Geometry: final body of the model. Coordinates: model frame, mm. Face numbers are marked on the shaded views. Give positions to 0.01 mm unless a question says otherwise; leave off trailing zeros. Order: outer loops, then holes, each group sorted by start corner. A loop starts at its lowest first (then second) coordinate and runs counter-clockwise, first axis right, second up. Notation, with made-up numbers: (-32.75, -19.75) -> (-28.75, -19.75) arc R15 cw to (-28.75, -10.75) -> close; hole circle Ø3 at (-17.75, 76.5). An arc over 180 degrees is marked (long way). Answer in a Markdown table with one row per item. Add a question column.
Q1. Line query: line 1 along X through (y, z) = (0, 3.25); line 2 along X through (y, z) = (-1, 5.5); line 3 along Y through (x, z) = (-4.25, -0.75). Output: solid intervals per line, ascending. Write a range as from..to.
Q2. Pull-direction query (X, two-part tool) for the marked faces 1, 2, 3 and 4; classes: +X half, -X half, draft (parallel to the pull), parting line (faces both ways), or undercut.
Q3. Cut plane A-A on z = 1.5. Return the cut outline in (x, y), and give its area (3 significant figures).
Q4. Contact query for flat-ended pins moving along their axis: P1, Ø5, axis at x = -3, z = -3, coming from the +Y side; P2, Ø3, axis at x = 0.5, z = 0.5, coming from the +Y side; P3, Ø7, axis at x = 0, y = 0, coming from the -Z side. Output: stop coordinate, or through.
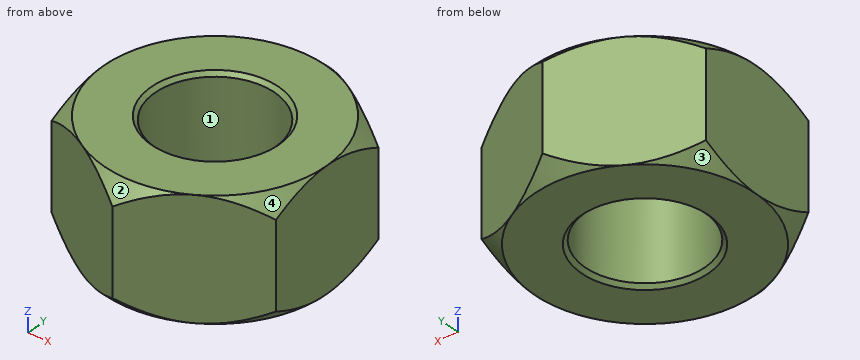
from build123d import *

# Parameters (mm, degrees)
SKETCH1_R           = 6
BOSS_EXTRUDE1_DEPTH = 6
SKETCH6_OUTSIDE_W   = 74.94
SKETCH6_OUTSIDE_H   = 78.374
SKETCH6_OUTSIDE_R   = 11.1
CUT_EXTRUDE5_DEPTH  = 21.772337374
CUT_EXTRUDE5_DRAFT  = -45
SKETCH7_OUTSIDE_W   = 74.94
SKETCH7_OUTSIDE_H   = 78.374
SKETCH7_OUTSIDE_R   = 11.1
CUT_EXTRUDE6_DEPTH  = 21.772337374
CUT_EXTRUDE6_DRAFT  = -45


with BuildPart() as part:
    # Sketch1 → Boss-Extrude1 (new, symmetric)
    with BuildSketch(Plane.XY):
        Polygon((0, -12.817175976), (11.1, -6.408587988), (11.1, 6.408587988), (0, 12.817175976), (-11.1, 6.408587988), (-11.1, -6.408587988), align=None)
        Circle(SKETCH1_R, mode=Mode.SUBTRACT)
    extrude(amount=BOSS_EXTRUDE1_DEPTH, both=True)

    # Cut-Extrude3 cone 1 section (through the dimple's axis) → Cut-Extrude3 (revolve, cut)
    with BuildSketch(Plane(origin=(0, 0, 6), x_dir=(0, -1, 0), z_dir=(1, 0, 0))):
        Polygon((0, 0), (6.381, 0), (0, 6.381), align=None)
    revolve(axis=Axis((0, 0, 6), (0, 0, -1)), mode=Mode.SUBTRACT)

    # Cut-Extrude4 cone 1 section (through the dimple's axis) → Cut-Extrude4 (revolve, cut)
    with BuildSketch(Plane(origin=(0, 0, -6), x_dir=(0, 1, 0), z_dir=(1, 0, 0))):
        Polygon((0, 0), (6.381, 0), (0, 6.381), align=None)
    revolve(axis=Axis((0, 0, -6), (0, 0, 1)), mode=Mode.SUBTRACT)


with BuildPart() as cut_extrude5_tool:
    # Sketch6 outside → Cut-Extrude5 (with draft: the straight prism first)
    with BuildSketch(Plane.XY.offset(6)):
        Rectangle(SKETCH6_OUTSIDE_W, SKETCH6_OUTSIDE_H)
        Circle(SKETCH6_OUTSIDE_R, mode=Mode.SUBTRACT)
    extrude(amount=-CUT_EXTRUDE5_DEPTH)
    # Cut-Extrude5: the draft: its side faces are tilted about the plane it starts from
    cut_extrude5_sides = [cut_extrude5_tool.faces().sort_by_distance(p)[0] for p in [
        (0, -39.187, -4.886168687),
        (37.47, 0, -4.886168687),
        (0, 39.187, -4.886168687),
        (-37.47, 0, -4.886168687),
        (-11.1, 0, -4.886168687),
    ]]
    draft(cut_extrude5_sides, Plane.XY.offset(6), CUT_EXTRUDE5_DRAFT)


with BuildPart() as part_1:
    add(part.part)

    # Cut-Extrude5: cut by cut_extrude5_tool
    add(cut_extrude5_tool.part, mode=Mode.SUBTRACT)


with BuildPart() as cut_extrude6_tool:
    # Sketch7 outside → Cut-Extrude6 (with draft: the straight prism first)
    with BuildSketch(Plane(origin=(0, 0, -6), x_dir=(-1, 0, 0), z_dir=(0, 0, -1))):
        Rectangle(SKETCH7_OUTSIDE_W, SKETCH7_OUTSIDE_H)
        Circle(SKETCH7_OUTSIDE_R, mode=Mode.SUBTRACT)
    extrude(amount=-CUT_EXTRUDE6_DEPTH)
    # Cut-Extrude6: the draft: its side faces are tilted about the plane it starts from
    cut_extrude6_sides = [cut_extrude6_tool.faces().sort_by_distance(p)[0] for p in [
        (0, -39.187, 4.886168687),
        (-37.47, 0, 4.886168687),
        (0, 39.187, 4.886168687),
        (37.47, 0, 4.886168687),
        (11.1, 0, 4.886168687),
    ]]
    draft(cut_extrude6_sides, Plane(origin=(0, 0, -6), x_dir=(-1, 0, 0), z_dir=(0, 0, -1)), CUT_EXTRUDE6_DRAFT)


with BuildPart() as part_2:
    add(part_1.part)

    # Cut-Extrude6: cut by cut_extrude6_tool
    add(cut_extrude6_tool.part, mode=Mode.SUBTRACT)


solid = part_2.part
Completed:
| question | item | result |
|---|---|---|
| 1 | line 1 | x = -11.1..-6, 6..11.1 |
| 1 | line 2 | x = -11.1..-5.92, 5.92..11.1 |
| 1 | line 3 | y = -10.36..-4.24, 4.24..10.36 |
| 2 | face 1 | undercut |
| 2 | face 2 | parting line |
| 2 | face 3 | -X half |
| 2 | face 4 | +X half |
| 3 | outline | (-11.1, -6.41) -> (0, -12.82) -> (11.1, -6.41) -> (11.1, 6.41) -> (0, 12.82) -> (-11.1, 6.41) -> close; hole circle Ø12 at (0, 0) |
| 3 | area | 314 mm² |
| 4 | P1 | stops at y = 12.53 |
| 4 | P2 | stops at y = 12.82 |
| 4 | P3 | passes through |
